from build123d import *

# Parameters (mm, degrees)
SKETCH_1_W          = 14.12
SKETCH_1_H          = 9.9
EXTRUDE_1_DEPTH     = 5.4
SKETCH_2_R          = 0.075
EXTRUDE_2_DEPTH     = 1.6
SKETCH_3_W          = 0.5
SKETCH_3_H          = 4
CUT_EXTRUDE_1_DEPTH = 4
SKETCH_4_W          = 1.5
SKETCH_4_H          = 4
CUT_EXTRUDE_2_DEPTH = 1
SKETCH_5_W          = 1.3
SKETCH_5_H          = 1.3
EXTRUDE_3_DEPTH     = 2


with BuildPart() as part:
    # 草图1 → 凸台-拉伸1 (new body)
    with BuildSketch(Plane(origin=(0, 0, 0), x_dir=(1, 0, 0), z_dir=(0, 1, 0))):
        with Locations((7.06, 4.95)):
            Rectangle(SKETCH_1_W, SKETCH_1_H)
    extrude(amount=EXTRUDE_1_DEPTH)

    # 草图2 → 凸台-拉伸2 (add)
    with BuildSketch(Plane.XZ):
        with Locations((1.98, -1.14)):
            Circle(SKETCH_2_R)
        with Locations((4.52, -1.14)):
            Circle(SKETCH_2_R)
        with Locations((7.06, -1.14)):
            Circle(SKETCH_2_R)
        with Locations((9.6, -1.14)):
            Circle(SKETCH_2_R)
        with Locations((12.14, -1.14)):
            Circle(SKETCH_2_R)
        with Locations((4.52, -8.76)):
            Circle(SKETCH_2_R)
        with Locations((7.06, -8.76)):
            Circle(SKETCH_2_R)
        with Locations((9.6, -8.76)):
            Circle(SKETCH_2_R)
        with Locations((12.14, -8.76)):
            Circle(SKETCH_2_R)
        with Locations((1.98, -8.76)):
            Circle(SKETCH_2_R)
    extrude(amount=EXTRUDE_2_DEPTH)

    # 草图3 → 切除-拉伸1 (cut)
    with BuildSketch(Plane(origin=(0, 5.4, 0), x_dir=(1, 0, 0), z_dir=(0, 1, 0))):
        with Locations((0.25, 4.95)):
            Rectangle(SKETCH_3_W, SKETCH_3_H)
    extrude(amount=-CUT_EXTRUDE_1_DEPTH, mode=Mode.SUBTRACT)

    # 草图4 → 切除-拉伸2 (cut)
    with BuildSketch(Plane(origin=(0, 5.4, 0), x_dir=(1, 0, 0), z_dir=(0, 1, 0))):
        with Locations((4.45, 4.95)):
            Rectangle(SKETCH_4_W, SKETCH_4_H)
        with Locations((1.75, 4.95)):
            Rectangle(SKETCH_4_W, SKETCH_4_H)
        with Locations((7.15, 4.95)):
            Rectangle(SKETCH_4_W, SKETCH_4_H)
        with Locations((9.85, 4.95)):
            Rectangle(SKETCH_4_W, SKETCH_4_H)
        with Locations((12.55, 4.95)):
            Rectangle(SKETCH_4_W, SKETCH_4_H)
    extrude(amount=-CUT_EXTRUDE_2_DEPTH, mode=Mode.SUBTRACT)

    # 草图5 → 凸台-拉伸3 (add)
    with BuildSketch(Plane(origin=(0, 4.4, 0), x_dir=(1, 0, 0), z_dir=(0, 1, 0))):
        with Locations((4.45, 3.65)):
            Rectangle(SKETCH_5_W, SKETCH_5_H)
        with Locations((1.75, 3.65)):
            Rectangle(SKETCH_5_W, SKETCH_5_H)
        with Locations((7.15, 3.65)):
            Rectangle(SKETCH_5_W, SKETCH_5_H)
        with Locations((9.85, 3.65)):
            Rectangle(SKETCH_5_W, SKETCH_5_H)
        with Locations((12.55, 3.65)):
            Rectangle(SKETCH_5_W, SKETCH_5_H)
    extrude(amount=EXTRUDE_3_DEPTH)


solid = part.part
Verification items for the finished model (mm, model axes). A direction names the side the tool comes from. Coordinates: 2 decimals unless noted, no trailing zeros. Order: outer loops, then holes, each group sorted by start corner. A loop starts at its lowest first (then second) coordinate and runs counter-clockwise, first axis right, second up. Notation, with made-up numbers: M 41.5,-11.75 L 86.5,-11.75 A21 ccw 86.5,10.25 Z; hole C 77.25,59 d7. An arc over 180 degrees is marked long. One line per item, written item: value. Start each with the question number.
Item 1: Gauge pin test, flat ends, axial feed: pin 1 (3 mm diameter, centred on x = 4, z = -5, fed in from +Y); pin 2 (1.6 mm diameter, centred on x = 1.5, z = -6, fed in from +Y); pin 3 (2 mm diameter, centred on x = 9.5, z = -5, fed in from -Y); pin 4 (0.5 mm diameter, centred on y = 5, z = -4.5, fed in from -X). Record the tip position at first contact, or that the pin passes through.
Item 2: Scan lines: probe 1 along Y at (x, z) = (10.25, -5.75); probe 2 along Y at (x, z) = (3, -7.5); probe 3 along Z at (x, y) = (10, 5.5). Record each from-to range of solid material in increasing order.
Item 3: Access from +Z, -Z, +X, -X, +Y, -Y to the whole of each face (thin tool, end or side, straight path). Record for faces 1 (the flat face through (4, 6.4, -4)), 2 (the flat face through (2.5, 5, -5)).
Item 4: Sectioned sample at A-A (z = -4.75). Enter the section's corners in (x, y), then the cut area to 3 significant figures.
Item 5: Mould release check, pull along Z, two halves, no side actions. Record for faces 3 (the flat face through (7, 3, 0)), 4 (the flat face through (7, 6.4, -4)), 5 (the flat face through (13, 6, -3)), 6 (the flat face through (7, 3, -9.9)): released by +Z, released by -Z, zero draft, split by the parting line, or undercut.
Item 6: Sectioned sample at C-C (z = -8). Enter the section's corners in (x, y).
Item 7: Sectioned sample at B-B (x = 6). Enter the section's corners in (y, z), then the cut area to 3 significant figures.
Conclusion:
1. pin 1: stops at y = 6.4
1. pin 2: stops at y = 5.4
1. pin 3: stops at y = 0
1. pin 4: stops at x = 0.5
2. probe 1: y = 0 to 4.4
2. probe 2: y = 0 to 5.4
2. probe 3: z = -4.3 to -3
3. face 1: +Z, -Z, +X, -X, +Y
3. face 2: +Y
4. outline: M 0,0 L 14.12,0 L 14.12,5.4 L 13.3,5.4 L 13.3,4.4 L 11.8,4.4 L 11.8,5.4 L 10.6,5.4 L 10.6,4.4 L 9.1,4.4 L 9.1,5.4 L 7.9,5.4 L 7.9,4.4 L 6.4,4.4 L 6.4,5.4 L 5.2,5.4 L 5.2,4.4 L 3.7,4.4 L 3.7,5.4 L 2.5,5.4 L 2.5,4.4 L 1,4.4 L 1,5.4 L 0.5,5.4 L 0.5,1.4 L 0,1.4 Z
4. area: 66.7 mm^2
5. face 3: released by +Z
5. face 4: zero draft
5. face 5: undercut
5. face 6: released by -Z
6. outline: M 0,0 L 14.12,0 L 14.12,5.4 L 0,5.4 Z
7. outline: M 0,-9.9 L 5.4,-9.9 L 5.4,0 L 0,0 Z
7. area: 53.5 mm^2
